Here's how the part is built. I have some questions about the finished solid (model axes, mm). Face numbers are marked on the shaded views. A direction names the side the tool comes from. Round coordinates to 2 decimals unless told otherwise and drop trailing zeros. Write item = value, one per line. Start each with the question number.
(1) Will these pins go through, and if not, where does the flat tip stop? pin 1 Ø8 at (x, y) = (14.5, 14) entering from +Z; pin 2 Ø10 at (x, y) = (-6, 61.5) entering from +Z; pin 3 Ø4 at (y, z) = (42.5, -33.5) entering from -X.
(2) If we mould it in two halves opening along X, with no side actions, what happens to the marked faces 1 and 2? For each: released by +X, released by -X, zero draft, split by the parting line, or undercut.
(3) I need wall thicknesses on line 1 along X through (y, z) = (50.5, 55); line 2 along Z through (x, y) = (60.5, 61); line 3 along X through (y, z) = (81.5, 44.5). Which ranges of each line are inside material? Lowest first, please.
(4) On a 3-axis mill with a long thin cutter (end or side, diameter ignored), from which of +Z, -Z, +X, -X, +Y, -Y can I reach the whole of each face in a straight line? I mean the marked faces 3 and 4. Say none if no direction works.
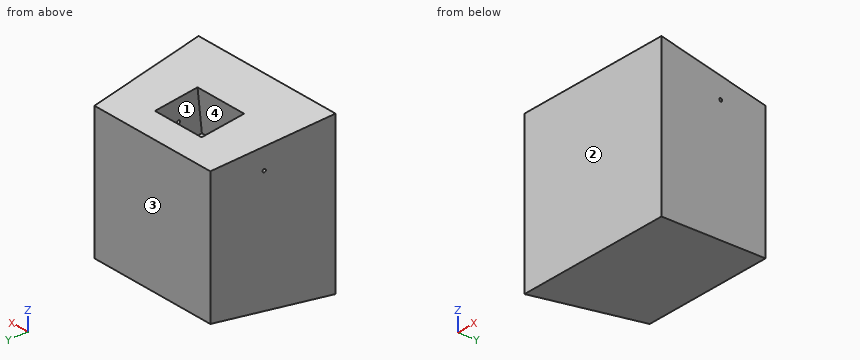
```python
from build123d import *

# Parameters (mm, degrees)
SKETCH1_W               = 150
SKETCH1_H               = 150
BOSS_EXTRUDE1_DEPTH     = 110
BOSS_EXTRUDE1_TAPER     = 6
SKETCH14_W              = 51
SKETCH14_H              = 41
CUT_EXTRUDE2_DEPTH      = 40
CUT_EXTRUDE3_DEPTH      = 167.809022709
CUT_EXTRUDE3_DEPTH_BACK = 167.809022709
SKETCH23_R              = 1.5


with BuildPart() as part:
    # Sketch1 → Boss-Extrude1 (new body)
    with BuildSketch(Plane(origin=(0, 0, 0), x_dir=(1, 0, 0), z_dir=(0, 1, 0))):
        Rectangle(SKETCH1_W, SKETCH1_H)
    extrude(amount=BOSS_EXTRUDE1_DEPTH, taper=BOSS_EXTRUDE1_TAPER)

    # Sketch14 → Cut-Extrude2 (cut)
    with BuildSketch(Plane(origin=(0, 7.796688406, 74.180535028), x_dir=(1, 0, 0), z_dir=(0, 0.10452846326765353, 0.9945218953682734))):
        with Locations((0, 57.266276007)):
            Rectangle(SKETCH14_W, SKETCH14_H)
    extrude(amount=-CUT_EXTRUDE2_DEPTH, mode=Mode.SUBTRACT)

    # Sketch23 → Cut-Extrude3 (cut, two sides: drawn at the far end of the back side and taken through both)
    with BuildSketch(Plane(origin=(-25.5, 0, 0), x_dir=(0, 0, -1), z_dir=(1, 0, 0)).offset(-CUT_EXTRUDE3_DEPTH_BACK)):
        with Locations(Location((-48.304141292, 62.658684495, 0), (0, 0, 90))):
            Circle(SKETCH23_R)
    extrude(amount=CUT_EXTRUDE3_DEPTH + CUT_EXTRUDE3_DEPTH_BACK, mode=Mode.SUBTRACT)


solid = part.part
```
Returned:
q1.pin_1 = 73.95
q1.pin_2 = 28.84
q1.pin_3 = -70.74
q2.face_1 = undercut
q2.face_2 = zero draft
q3.line_1 = -69.69 to -25.5, 25.5 to 69.69
q3.line_2 = -68.59 to 68.59
q3.line_3 = -66.43 to -25.5, 25.5 to 66.43
q4.face_3 = +Z, -Z, +X, -X, +Y
q4.face_4 = none
